For this review, use the dimensioned drawing (mm, ordinates from the lowest corner) and the shaded views. A direction names the side the tool comes from. Coordinates: 2 decimals unless noted, no trailing zeros. Write each loop counter-clockwise with the first axis right and the second up, starting at its lowest first coordinate (ties: lowest second). Pieces come first, ordered by that corner, then holes. Notation, with made-up numbers: (-18.5, -6) -> (30.5, -6) arc R12 cw to (30.5, 12) -> close; hole circle Ø11 at (88, 72.5). An arc over 180 degrees is marked (long way). Put each result on its own line as item: value. Start each with the question number.
Item 1: To check wall thickness, follow L1, parallel to X at y = 18, z = 41.5; L2, parallel to Z at x = 14, y = 9.25; L3, parallel to Y at x = 18.75, z = 43.5. State the ranges of each line that lie inside material, in increasing order.
Item 2: Consider section C-C on z = 30. Give the boundary of the cut face in (x, y), and give its area (3 significant figures).
Item 3: Consider section D-D on y = 8.75. Give the boundary of the cut face in (x, z), and give its area (3 significant figures).
Item 4: Consider section A-A on y = 19.5. Give the boundary of the cut face in (x, z).
Item 5: Insertion check: P1, Ø1.5, axis at y = 23.5, z = 37.5, coming from the -X side; P2, Ø9.5, axis at x = 10, z = 37.5, coming from the -Y side; P3, Ø1.5, axis at y = 23.5, z = 22, coming from the +X side. Each pin has a flat end and moves straight along its axis. Give the tip position at first contact, or say it passes through.
Item 6: Consider section B-B on x = 10.75. Give the boundary of the cut face in (y, z).
Item 7: For the marked faces 1, 2, 3 and 4, list the 3-axis set-ups (+Z, -Z, +X, -X, +Y, -Y) from which the entire face can be reached by the end or side of a thin tool; tool diameter is ignored.
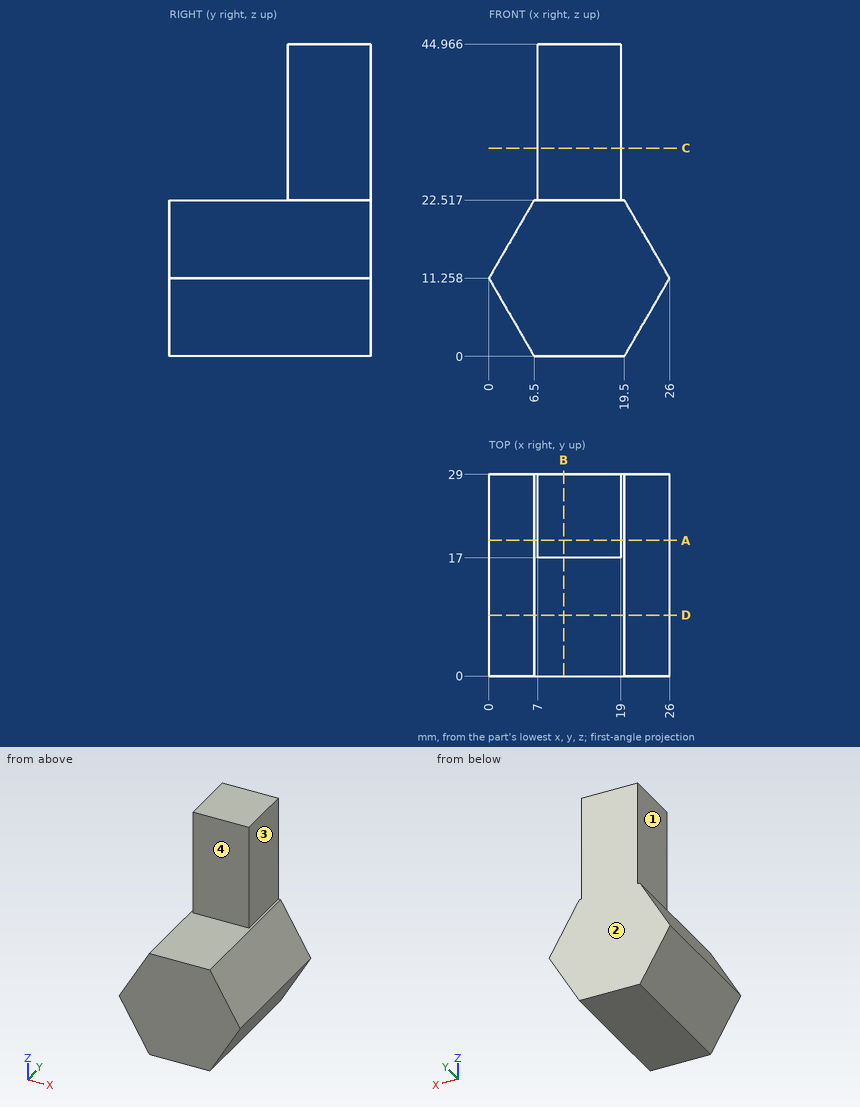
Return value:
1. L1: 7 to 19
1. L2: 0 to 22.52
1. L3: 17 to 29
2. outline: (7, 17) -> (19, 17) -> (19, 29) -> (7, 29) -> close
2. area: 144 mm^2
3. outline: (0, 11.26) -> (6.5, 0) -> (19.5, 0) -> (26, 11.26) -> (19.5, 22.52) -> (6.5, 22.52) -> close
3. area: 439 mm^2
4. outline: (0, 11.26) -> (6.5, 0) -> (19.5, 0) -> (26, 11.26) -> (19.5, 22.52) -> (19, 22.52) -> (19, 44.97) -> (7, 44.97) -> (7, 22.52) -> (6.5, 22.52) -> close
5. P1: x = 7
5. P2: y = 17
5. P3: x = 20.23
6. outline: (0, 0) -> (29, 0) -> (29, 44.97) -> (17, 44.97) -> (17, 22.52) -> (0, 22.52) -> close
7. face 1: +Z, -X, +Y, -Y
7. face 2: +Z, -Z, +X, -X, +Y
7. face 3: +Z, +X, +Y, -Y
7. face 4: +Z, +X, -X, -Y
